Source: three-view drawing plus pictorial views. Frame: mm from the lowest corner of the part. A direction names the side the tool comes from. Give positions to 0.01 mm unless a question says otherwise; leave off trailing zeros. Loops run counter-clockwise (first coordinate to the right, second up) from the corner with the lowest first, then second, coordinate; pieces in that order, holes last. Notation, with made-up numbers: (-8, -9.75) - (3, -9.75) arc R30 ccw to (3, 17.25) - close; hole circle Ø5 at (-31.75, -11.75). An arc over 180 degrees is marked (long way). Answer as a JSON object with one key per item and string values.
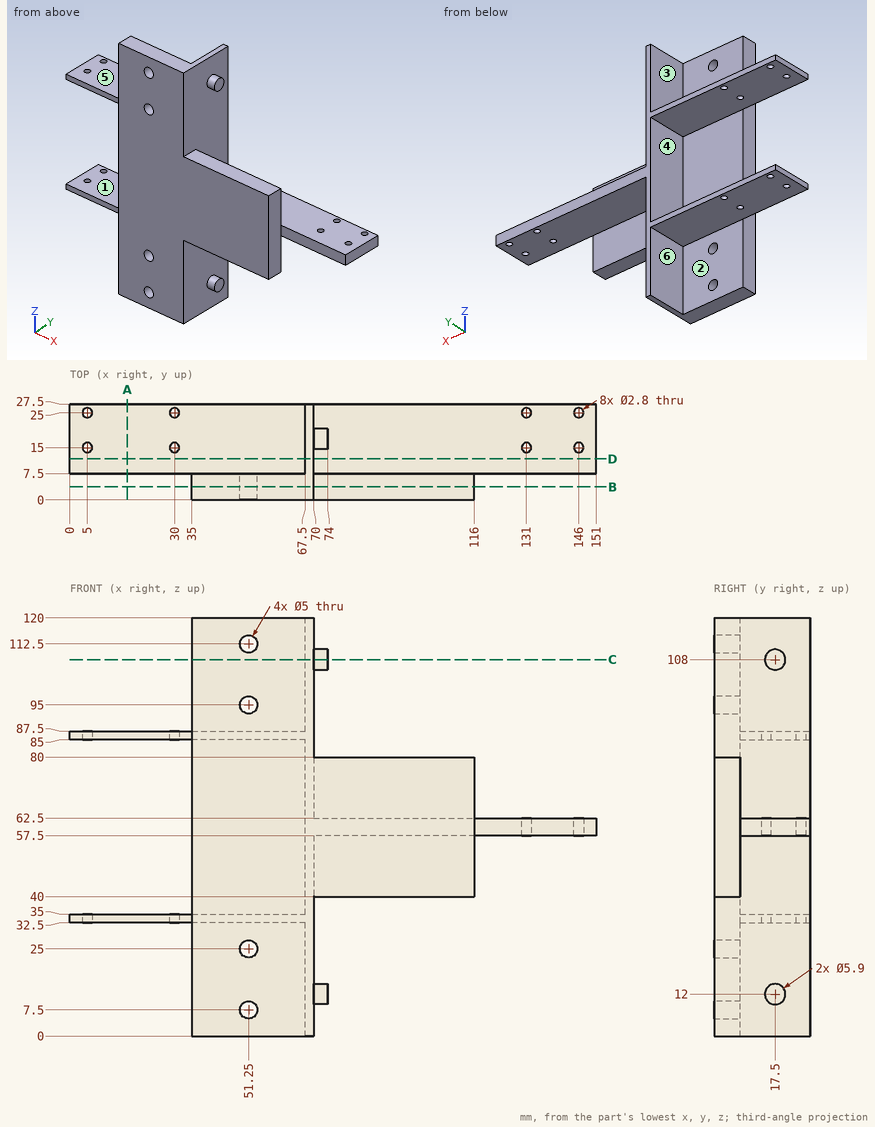
Item 1: Access query for the marked faces 1, 2 and 3. Directions: +Z, -Z, +X, -X, +Y, -Y. A direction counts if a zero-diameter tool reaches every point of the face in a straight line with its end or side. Return the directions, or none.
Geometry check:
{"face 1": "-X, +Y", "face 2": "-Z, -X, +Y", "face 3": "+Z, -X, +Y"}
Item 2: Cut plane B-B (y = 3.75). Return loops of the section in (x, z).
Geometry check:
{"outline": "(35, 0) - (70, 0) - (70, 40) - (116, 40) - (116, 80) - (70, 80) - (70, 120) - (35, 120) - close; hole circle Ø5 at (51.25, 7.5); hole circle Ø5 at (51.25, 25); hole circle Ø5 at (51.25, 95); hole circle Ø5 at (51.25, 112.5)"}
Item 3: Cut plane C-C (z = 108). Return loops of the section in (x, y), then the cut area to 3 significant figures.
Geometry check:
{"outline": "(35, 0) - (70, 0) - (70, 14.55) - (74, 14.55) - (74, 20.45) - (70, 20.45) - (70, 27.5) - (67.5, 27.5) - (67.5, 7.5) - (35, 7.5) - close", "area": "336 mm2"}
Item 4: Cut plane A-A (x = 16.5). Return loops of the section in (y, z), then the cut area to 3 significant figures.
Geometry check:
{"outline": "(7.5, 32.5) - (27.5, 32.5) - (27.5, 35) - (7.5, 35) - close; (7.5, 85) - (27.5, 85) - (27.5, 87.5) - (7.5, 87.5) - close", "area": "100 mm2"}
Item 5: Contact query for flat-ended pins moving along their axis: P1, Ø8, axis at x = 102.5, y = 19.5, coming from the +Z side; P2, Ø10, axis at x = 66, y = 23, coming from the -Z side; P3, Ø3.5, axis at x = 30, y = 25, coming from the -Z side; P4, Ø5, axis at x = 90.5, z = 53, coming from the +Y side. Output: stop coordinate, or through.
Geometry check:
{"P1": "stops at z = 62.5", "P2": "stops at z = 0", "P3": "stops at z = 32.5", "P4": "stops at y = 7.5"}
Item 6: Mould query, pull axis Z, two halves, no side actions, for the marked faces 4, 5 and 6. Classes: released by +Z, released by -Z, zero draft, split by the parting line, or undercut.
Geometry check:
{"face 4": "undercut", "face 5": "released by +Z", "face 6": "zero draft"}
Item 7: Cut plane D-D (y = 11.75). Return loops of the section in (x, z).
Geometry check:
{"outline": "(0, 32.5) - (67.5, 32.5) - (67.5, 0) - (70, 0) - (70, 57.5) - (151, 57.5) - (151, 62.5) - (70, 62.5) - (70, 120) - (67.5, 120) - (67.5, 87.5) - (0, 87.5) - (0, 85) - (67.5, 85) - (67.5, 35) - (0, 35) - close"}
Item 8: Material intervals for line 1 (Y direction, x = 30, z = 86); line 2 (Z direction, x = 17, y = 16.5); line 3 (X direction, y = 14.5, z = 85.5), sorted ascending. Write a range as [from, to].
Geometry check:
{"line 1": "y = [7.5, 13.6], [16.4, 23.6], [26.4, 27.5]", "line 2": "z = [32.5, 35], [85, 87.5]", "line 3": "x = [0, 3.69], [6.31, 28.69], [31.31, 70]"}
